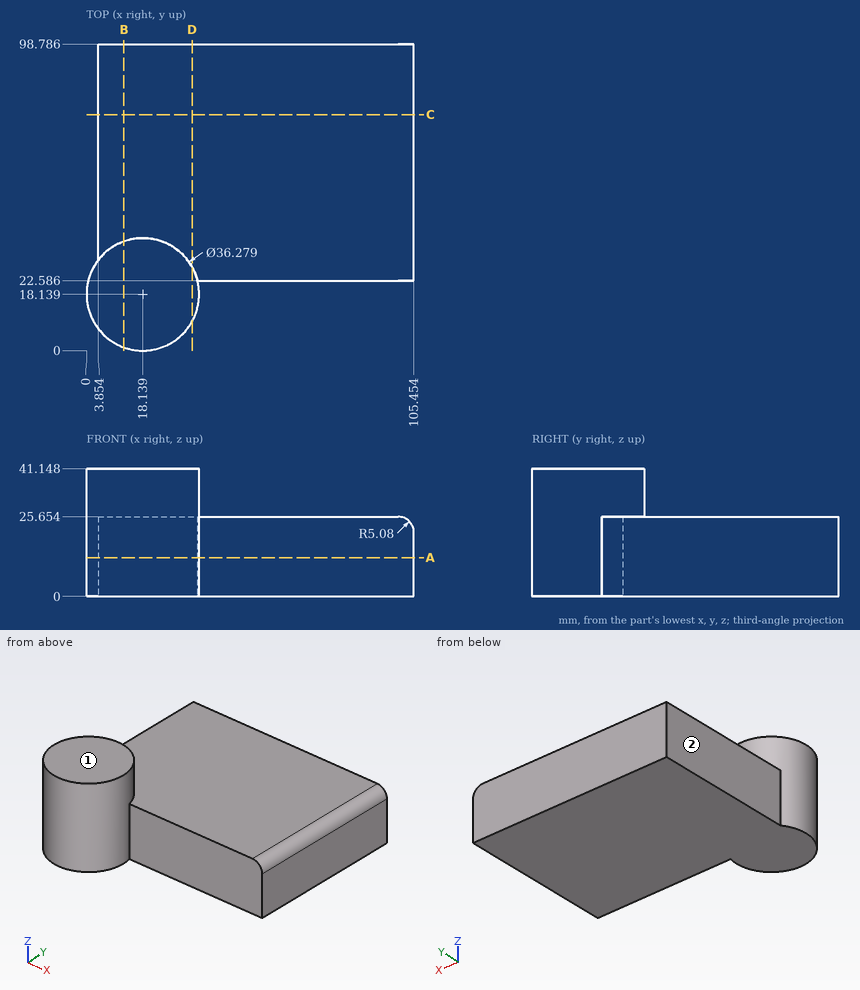
For this review, use the dimensioned drawing (mm, ordinates from the lowest corner) and the shaded views. A direction names the side the tool comes from. Give positions to 0.01 mm unless a question says otherwise; leave off trailing zeros. Write each loop counter-clockwise with the first axis right and the second up, starting at its lowest first coordinate (ties: lowest second). Pieces come first, ordered by that corner, then holes. Notation, with made-up numbers: M 33,68 L 38,68 A23 ccw 38,101 Z; hole C 14.25,34 d1. An arc over 180 degrees is marked long. Answer as a JSON object with one key per item and string values. Group by question number.
Item 1: For probe 1 along Z at (x, y) = (38.5, 53.5); probe 2 along Y at (x, z) = (66, 9.5); probe 3 along X at (y, z) = (30, 2), list the stretches that pass through material, from the lowest coordinate up. Write a range as [from, to].
Item 2: Consider section D-D on x = 34. Write out the cut boundary in (y, z), plus the area to 3 significant figures.
Item 3: For pin 1 Ø8 at (x, y) = (94, 84.5) entering from +Z; pin 2 Ø10 at (y, z) = (29.5, 36) entering from -X; pin 3 Ø7.5 at (y, z) = (70.5, 18) entering from -X, all flat-tipped, find the tip position at first contact; note any pin that passes through.
Item 4: Consider section C-C on y = 76. Write out the cut boundary in (x, z).
Item 5: Consider section B-B on x = 12. Write out the cut boundary in (y, z), plus the area to 3 significant figures.
Item 6: Tool access review of the marked faces 1 and 2: name each direction out of +Z, -Z, +X, -X, +Y, -Y from which nothing blocks a thin tool from reaching the whole face with its end or side.
Item 7: Consider section A-A on z = 12.5. Write out the cut boundary in (x, y) (1 decimal).
Check result:
{
 "1": {"probe 1": "z = [0, 25.65]", "probe 2": "y = [22.59, 98.79]", "probe 3": "x = [3.85, 105.45]"},
 "2": {"outline": "M 9.34,0 L 98.79,0 L 98.79,25.65 L 26.94,25.65 L 26.94,41.15 L 9.34,41.15 Z", "area": "2,570 mm^2"},
 "3": {"pin 1": "stops at z = 25.65", "pin 2": "stops at x = 1.15", "pin 3": "stops at x = 3.85"},
 "4": {"outline": "M 3.85,0 L 105.45,0 L 105.45,20.57 A5.08 ccw 100.37,25.65 L 3.85,25.65 Z"},
 "5": {"outline": "M 1.07,0 L 98.79,0 L 98.79,25.65 L 35.21,25.65 L 35.21,41.15 L 1.07,41.15 Z", "area": "3,040 mm^2"},
 "6": {"face 1": "+Z, +X, -X, +Y, -Y", "face 2": "+Z, -Z, -X, +Y"},
 "7": {"outline": "M 3.9,29.3 A18.1 ccw long 35.7,22.6 L 105.5,22.6 L 105.5,98.8 L 3.9,98.8 Z"}
}
